For this review, take the finished solid that the model builds, in its own axes (mm). Coordinates: 2 decimals unless noted, no trailing zeros. Order: outer loops, then holes, each group sorted by start corner. A loop starts at its lowest first (then second) coordinate and runs counter-clockwise, first axis right, second up. Notation, with made-up numbers: M -13,-34 L -5,-34 A29 ccw -5,5 Z; hole C 66.5,16 d9. An arc over 180 degrees is marked long. Use CSV: the item, a comma, the result in double quotes.
```python
from build123d import *

# Parameters (mm, degrees)
F0_R     = 25
F1_DEPTH = 25
F2_SIZE2 = 24.99999
F2_SIZE  = 24.99999
F3_W     = 55
F3_H     = 55
F4_DEPTH = 30


# Not quite as in the source:
# - a fillet or chamfer is up to 0.001 mm smaller than in the source, because OpenCascade refuses the exact size


with BuildPart() as f1:
    # F0 (on Top) → F1 (new body, symmetric)
    with BuildSketch(Plane.XY):
        Circle(F0_R)
    extrude(amount=F1_DEPTH, both=True)

    # F2 (size 25 and 25 in the source; OpenCascade refuses exactly that, so slightly less here)
    f2_edges = [f1.edges().sort_by_distance(p)[0] for p in [
        (-25, 0, 25),
        (-25, 0, -25),
    ]]
    chamfer(f2_edges, length=F2_SIZE, length2=F2_SIZE2)

    # F3 (on Right) → F4 (cut)
    with BuildSketch(Plane.YZ):
        Rectangle(F3_W, F3_H)
    extrude(amount=F4_DEPTH, mode=Mode.SUBTRACT)


solid = f1.part
```
Item 1: Add section B-B on z = 21.5. State the section outline as (x, y) points.
Solutions:
outline,"M 0,-3.5 L 0,3.5 A3.5 ccw Z"
Item 2: Add section A-A on z = 7.5. State the section outline as (x, y) points.
Solutions:
outline,"M 0,-17.5 L 0,17.5 A17.5 ccw Z"
Item 3: Clearance check with flat-ended pins moving along their axes: pin 1 Ø8 at (x, y) = (-12, 1.5) entering from -Z; pin 2 Ø4 at (x, y) = (-16.5, 11) entering from +Z; pin 3 Ø5 at (x, z) = (-12.5, 17) entering from -Y; pin 4 Ø1 at (x, y) = (-18, 17.5) entering from -Z. State where each tip first meets the part, or that it passes through.
Solutions:
pin 1,"z = -16.91"
pin 2,"z = 7.17"
pin 3,"through"
pin 4,"z = -0.4"
Item 4: To check wall thickness, follow line 1 along Y through (x, z) = (-13.75, 2); line 2 along X through (y, z) = (-3.5, 5); line 3 along Y through (x, z) = (-8.75, 12). State the ranges of each line that lie inside material, in increasing order. Write a range as [from, to].
Solutions:
line 1,"[-18.44, 18.44]"
line 2,"[-19.69, 0]"
line 3,"[-9.61, 9.61]"
